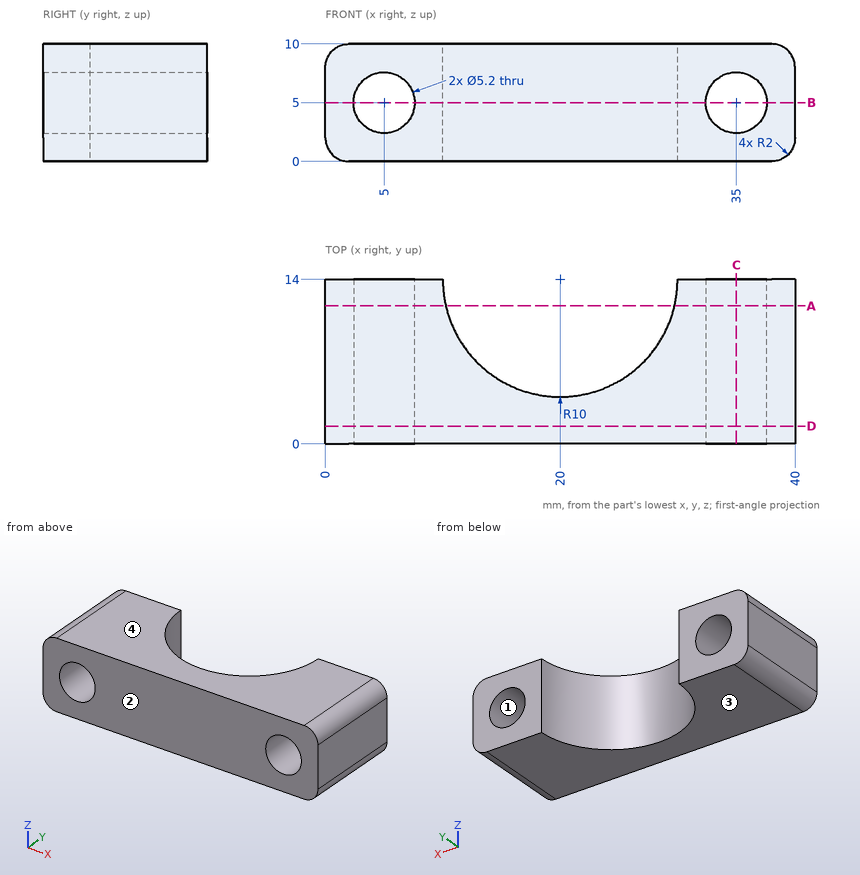
Geometry check sheet. Reference: drawing and pictorial views, mm from the part's lowest x, y, z. Coordinates: 2 decimals unless noted, no trailing zeros. Order: outer loops, then holes, each group sorted by start corner. A loop starts at its lowest first (then second) coordinate and runs counter-clockwise, first axis right, second up. Notation, with made-up numbers: M 32.25,66 L 85.25,66 A13 cw 85.25,74 Z; hole C 53.5,73 d4. An arc over 180 degrees is marked long. Write each question's results on one line, items separated by ' | '. Start each with the question number.
1. Go/stop test with a flat-tipped pin: P1, Ø1.5, axis at x = 22.5, z = 4.5, coming from the +Y side. Record where the tip stops, or that it passes through.
2. Cross-section at D-D on y = 1.5. Record the cut outline in (x, z), and give its area (3 significant figures).
3. Material ranges on probe 1 along X at (y, z) = (12.5, 7.25); probe 2 along X at (y, z) = (13.5, 5.25); probe 3 along Z at (x, y) = (35, 10.25), recorded low to high.
4. Cross-section at B-B on z = 5. Record the cut outline in (x, y), and give its area (3 significant figures).
5. Mould release check, pull along Z, two halves, no side actions. Record for the marked faces 1, 2, 3 and 4: +Z half, -Z half, draft (parallel to the pull), parting line (faces both ways), or undercut.
6. Cross-section at C-C on x = 35. Record the cut outline in (y, z), and give its area (3 significant figures).
7. Cross-section at A-A on y = 11.75. Record the cut outline in (x, z).
Checks:
1) P1: stops at y = 4.54
2) outline: M 0,2 A2 ccw 2,0 L 38,0 A2 ccw 40,2 L 40,8 A2 ccw 38,10 L 2,10 A2 ccw 0,8 Z; hole C 5,5 d5.2; hole C 35,5 d5.2 | area: 354 mm²
3) probe 1: x = 0 to 3.7, 6.3 to 10.11, 29.89 to 33.7, 36.3 to 40 | probe 2: x = 0 to 2.41, 7.59 to 10.01, 29.99 to 32.41, 37.59 to 40 | probe 3: z = 0 to 2.4, 7.6 to 10
4) outline: M 0,0 L 2.4,0 L 2.4,14 L 0,14 Z; M 7.6,0 L 32.4,0 L 32.4,14 L 30,14 A10 cw 10,14 L 7.6,14 Z; M 37.6,0 L 40,0 L 40,14 L 37.6,14 Z | area: 257 mm²
5) face 1: undercut | face 2: draft | face 3: -Z half | face 4: +Z half
6) outline: M 0,0 L 14,0 L 14,2.4 L 0,2.4 Z; M 0,7.6 L 14,7.6 L 14,10 L 0,10 Z | area: 67.2 mm²
7) outline: M 0,2 A2 ccw 2,0 L 10.26,0 L 10.26,10 L 2,10 A2 ccw 0,8 Z; M 29.74,0 L 38,0 A2 ccw 40,2 L 40,8 A2 ccw 38,10 L 29.74,10 Z; hole C 5,5 d5.2; hole C 35,5 d5.2
